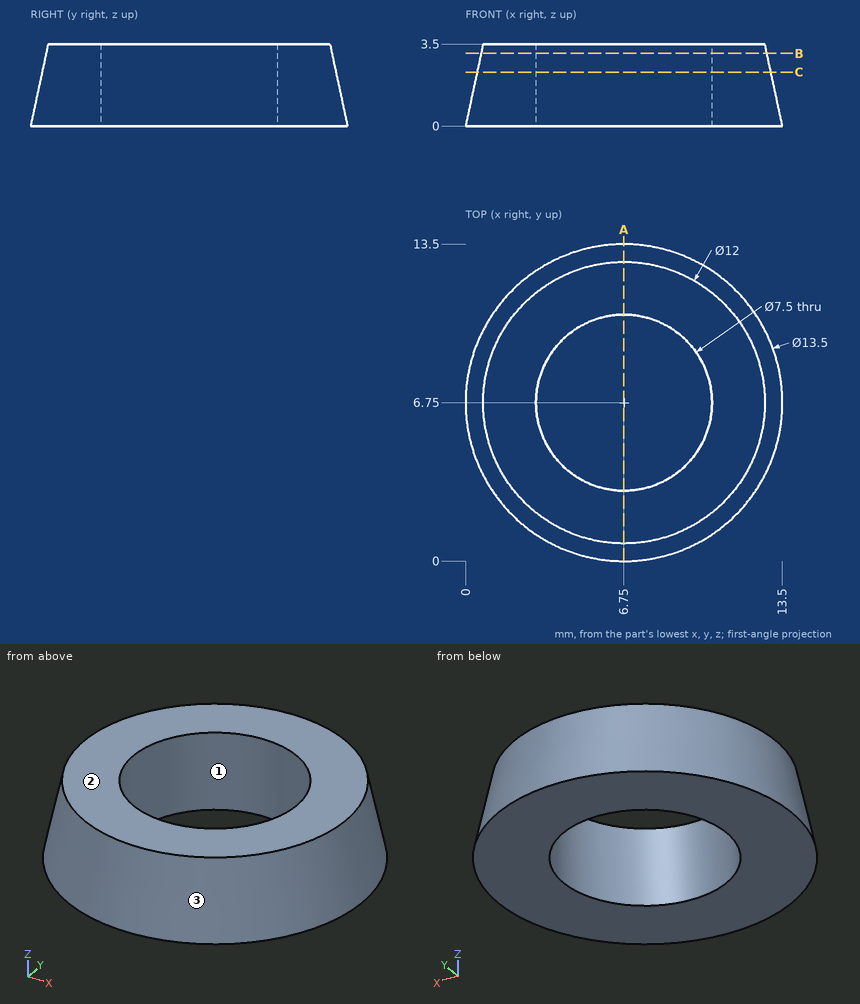
Can you work these out from the drawing? Everything is in mm from the part's minimum corner. Round coordinates to 2 decimals unless told otherwise and drop trailing zeros. Write each loop counter-clockwise with the first axis right and the second up, starting at its lowest first coordinate (ties: lowest second). Pieces come first, ordered by that corner, then holes.
1. Suppose I cut it at A-A (x = 6.75). List the corners of the cut face in (y, z) for me.
2. Will these pins go through, and if not, where does the flat tip stop? pin 1 Ø1 at (y, z) = (8.5, 2) entering from -X; pin 2 Ø2 at (y, z) = (2, 1.5) entering from +X; pin 3 Ø4.5 at (x, y) = (6.75, 6.75) entering from -Z.
3. Suppose I cut it at C-C (z = 2.3). List the corners of the cut face in (x, y) for me, and give its area (3 significant figures).
4. If we mould it in two halves opening along X, with no side actions, what happens to the marked faces 1, 2 and 3? For each: released by +X, released by -X, zero draft, split by the parting line, or undercut.
5. Suppose I cut it at B-B (z = 3.1). List the corners of the cut face in (x, y) for me.
6. I need wall thicknesses on L1, parallel to Y at x = 4, z = 2; L2, parallel to X at y = 7.25, z = 2.8; L3, parallel to X at y = 5.5, z = 2.5. Which ranges of each line are inside material? Lowest first, please.
Answer sheet:
1. outline: (0, 0) - (3, 0) - (3, 3.5) - (0.75, 3.5) - close; (10.5, 0) - (13.5, 0) - (12.75, 3.5) - (10.5, 3.5) - close
2. pin 1: stops at x = 0.51
2. pin 2: stops at x = 12.02
2. pin 3: passes through
3. outline: circle Ø12.51 at (6.75, 6.75); hole circle Ø7.5 at (6.75, 6.75)
3. area: 78.8 mm2
4. face 1: undercut
4. face 2: zero draft
4. face 3: split by the parting line
5. outline: circle Ø12.17 at (6.75, 6.75); hole circle Ø7.5 at (6.75, 6.75)
6. L1: y = 1.06 to 4.2, 9.3 to 12.44
6. L2: x = 0.62 to 3.03, 10.47 to 12.88
6. L3: x = 0.66 to 3.21, 10.29 to 12.84
